The model under review builds one solid part; all positions refer to its coordinate system, in mm. Face numbers are marked on the shaded views. Round coordinates to 2 decimals unless told otherwise and drop trailing zeros. Write each loop counter-clockwise with the first axis right and the second up, starting at its lowest first coordinate (ties: lowest second). Pieces come first, ordered by that corner, then holes. Notation, with made-up numbers: M 21,52.5 L 59,52.5 A14 ccw 59,67.5 Z; hole C 49.5,16.5 d2. An arc over 180 degrees is marked long. One line per item, written item: value. Start each with the question number.
1) Wall thickness on probe 1 along Y at (x, z) = (0, 35.5); probe 2 along X at (y, z) = (12, 42); probe 3 along Y at (x, z) = (1, 42.5): over which ranges is each line inside the solid? List them lowest first.
2) For P1, Ø1, axis at x = -1, y = -39, coming from the -Z side; P2, Ø2.5, axis at x = 8.65, y = 12.5, coming from the +Z side; P3, Ø5, axis at y = -16.5, z = 15, coming from the -X side; P4, Ø3, axis at x = 38, z = 5, coming from the +Y side, all flat-tipped, find the tip position at first contact; note any pin that passes through.
3) Take a section at B-B, the plane y = 40. Write out the cut boundary in (x, z), and give its area (3 significant figures).
4) Take a section at A-A, the plane x = 0. Write out the cut boundary in (y, z), and give its area (3 significant figures).
5) Take a section at C-C, the plane y = -20. Write out the cut boundary in (x, z), and give its area (3 significant figures).
6) Take a section at D-D, the plane z = 12. Write out the cut boundary in (x, y), and give its area (3 significant figures).
7) Mouldability with a two-part tool opening along X and no side actions: class the marked faces 1, 2 and 3 as +X half, -X half, draft (parallel to the pull), parting line (faces both ways), or undercut.
from build123d import *

# Parameters (mm, degrees)
SKETCH1_R           = 50
BOSS_EXTRUDE1_DEPTH = 50
SKETCH2_R           = 3
CUT_EXTRUDE1_DEPTH  = 87.602540378
SKETCH6_R           = 1.5
CUT_EXTRUDE2_DEPTH  = 10
SKETCH7_R           = 7.5
CUT_EXTRUDE3_DEPTH  = 87.602540378


with BuildPart() as part:
    # Sketch1 → Boss-Extrude1 (new body)
    with BuildSketch(Plane.XY):
        Circle(SKETCH1_R)
    extrude(amount=BOSS_EXTRUDE1_DEPTH)

    # Sketch2 → Cut-Extrude1 (cut, through all)
    with BuildSketch(Plane.XY.offset(50)):
        with Locations((0, 40)):
            Circle(SKETCH2_R)
        with Locations((34.641016151, -20)):
            Circle(SKETCH2_R)
        with Locations((-34.641016151, -20)):
            Circle(SKETCH2_R)
        Circle(SKETCH2_R)
    extrude(amount=-CUT_EXTRUDE1_DEPTH, mode=Mode.SUBTRACT)

    # Sketch6 → Cut-Extrude2 (cut)
    with BuildSketch(Plane.XY.offset(50)):
        with Locations((21.650635095, 25.5)):
            Circle(SKETCH6_R)
        with Locations((34.650635095, 12.5)):
            Circle(SKETCH6_R)
        with Locations((21.650635095, -0.5)):
            Circle(SKETCH6_R)
        with Locations((8.650635095, 12.5)):
            Circle(SKETCH6_R)
    extrude(amount=-CUT_EXTRUDE2_DEPTH, mode=Mode.SUBTRACT)

    # Sketch7 → Cut-Extrude3 (cut, through all)
    with BuildSketch(Plane.XY.offset(50)):
        with Locations((15.556349186, -15.556349186)):
            Circle(SKETCH7_R)
    extrude(amount=-CUT_EXTRUDE3_DEPTH, mode=Mode.SUBTRACT)


solid = part.part
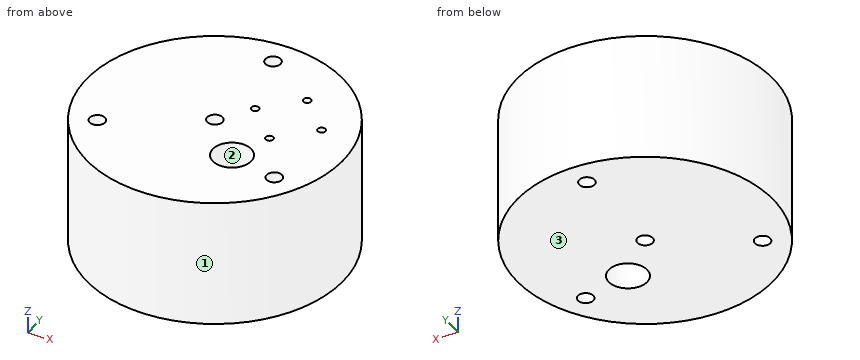
Checked values:
1. probe 1: y = -50 to -3, 3 to 37, 43 to 50
1. probe 2: x = -48.54 to 7.24, 10.06 to 33.24, 36.06 to 48.54
1. probe 3: y = -49.99 to -2.83, 2.83 to 37.17, 42.83 to 49.99
2. P1: stops at z = 0
2. P2: stops at z = 40
2. P3: stops at x = -48
2. P4: stops at y = 34.17
3. outline: M -30,0 L -3,0 L -3,50 L -30,50 Z; M 3,0 L 30,0 L 30,50 L 3,50 Z
3. area: 2,700 mm2
4. outline: M -50,0 L -3,0 L -3,50 L -50,50 Z; M 3,0 L 37,0 L 37,50 L 3,50 Z; M 43,0 L 50,0 L 50,50 L 43,50 Z
4. area: 4,400 mm2
5. outline: M -45.83,0 L -37.64,0 L -37.64,50 L -45.83,50 Z; M -31.64,0 L 9.51,0 L 9.51,50 L -31.64,50 Z; M 21.6,0 L 31.64,0 L 31.64,50 L 21.6,50 Z; M 37.64,0 L 45.83,0 L 45.83,50 L 37.64,50 Z
5. area: 3,380 mm2
6. outline: C 0,0 d100; hole C -34.64,-20 d6; hole C 0,0 d6; hole C 0,40 d6; hole C 15.56,-15.56 d15; hole C 34.64,-20 d6
6. area: 7,560 mm2
7. face 1: parting line
7. face 2: undercut
7. face 3: draft
